For this review, take the finished solid that the model builds, in its own axes (mm). A direction names the side the tool comes from. Coordinates: 2 decimals unless noted, no trailing zeros. Loops run counter-clockwise (first coordinate to the right, second up) from the corner with the lowest first, then second, coordinate; pieces in that order, holes last. Notation, with made-up numbers: (-14, -35.75) -> (37, -35.75) arc R30 ccw to (37, -8.75) -> close; hole circle Ø4 at (16.25, 22.5). An arc over 180 degrees is marked (long way). One line per item, written item: value.
from build123d import *

# Parameters (mm, degrees)
SKETCH2_R                     = 4.7625
LOCATION_START                = -5.08
SKETCH4_R                     = 1.524
LOCATION_HOLE_OTHER_WAY_DEPTH = 81.074387678


with BuildPart() as part:
    # Handle: sweep along a path in Sketch3
    with BuildLine(Plane(origin=(0, 0, 0), x_dir=(1, 0, 0), z_dir=(0, 1, 0))) as handle_path:
        Line((62.70625, 19.05), (62.70625, -2.3495))
        ThreePointArc((62.70625, -2.3495), (57.814786799, -14.158536799), (46.00575, -19.05))
        Line((46.00575, -19.05), (-46.00575, -19.05))
        ThreePointArc((-46.00575, -19.05), (-57.814786799, -14.158536799), (-62.70625, -2.3495))
        Line((-62.70625, -2.3495), (-62.70625, 19.05))
    # Sketch2 → Handle (sweep)
    with BuildSketch(Plane.XY.offset(-19.05)):
        with Locations((-62.70625, 0)):
            Circle(SKETCH2_R)
    sweep(path=handle_path.line)

    # Location Hole cone 1 section (through the dimple's axis) → Location Hole (revolve, cut)
    with BuildSketch(Plane(origin=(-62.70625, 0, -13.97), x_dir=(0, 1, 0), z_dir=(1, 0, 0))):
        Polygon((0, 0), (1.524, 0), (0, 0.87988181), align=None)
    revolve(axis=Axis((-62.70625, 0, -13.97), (0, 0, 1)), mode=Mode.SUBTRACT)

    # Location Hole cone 2 section (through the dimple's axis) → Location Hole cone 2 (revolve, cut)
    with BuildSketch(Plane(origin=(62.70625, 0, -13.97), x_dir=(0, 1, 0), z_dir=(1, 0, 0))):
        Polygon((0, 0), (1.524, 0), (0, 0.87988181), align=None)
    revolve(axis=Axis((62.70625, 0, -13.97), (0, 0, 1)), mode=Mode.SUBTRACT)

    # Sketch4 → Location Hole other way (cut)
    with BuildSketch(Plane(origin=(0, 0, -19.05), x_dir=(-1, 0, 0), z_dir=(0, 0, -1)).offset(LOCATION_START)):
        with Locations((62.70625, 0)):
            Circle(SKETCH4_R)
        with Locations((-62.70625, 0)):
            Circle(SKETCH4_R)
    extrude(amount=LOCATION_HOLE_OTHER_WAY_DEPTH, mode=Mode.SUBTRACT)


solid = part.part
1. Insertion check: pin 1 Ø12 at (x, z) = (-21, 17.5) entering from -Y; pin 2 Ø4 at (x, y) = (62.71, 0) entering from +Z; pin 3 Ø3 at (y, z) = (-1, 18) entering from -X; pin 4 Ø4 at (y, z) = (-3, 15.5) entering from -X. Each pin has a flat end and moves straight along its axis. Give the tip position at first contact, or say it passes through.
Return value:
pin 1: stops at y = -4.76
pin 2: stops at z = 17.98
pin 3: stops at x = -62.05
pin 4: stops at x = -63.68
2. The part is to be moulded in two halves that separate along X. For faces 4 (the cylindrical face through (58.164, -1.431, -8.2)), 5 (the flat face through (-63, -2, -19.05)), say which applies: pulls with the +X half, pulls with the -X half, needs draft (parallel to the pull), parting line crosses it, or undercut.
Return value:
face 4: undercut
face 5: needs draft
3. To check wall thickness, follow probe 1 along X at (y, z) = (0, -17.25); probe 2 along X at (y, z) = (-0.5, -14); probe 3 along X at (y, z) = (3.5, -8). State the ranges of each line that lie inside material, in increasing order. Write a range as from..to.
Return value:
probe 1: x = -67.47..-64.23, -61.18..-57.94, 57.94..61.18, 64.23..67.47
probe 2: x = -67.44..-64.15, -61.27..-57.97, 57.97..61.27, 64.15..67.44
probe 3: x = -65.94..-59.48, 59.48..65.94
4. For faces 1 (the flat face through (63, -2, -19.05)), 2 (the cylindrical face through (-0.6, -1.4, 14.5)), 3 (the cylindrical face through (-58.164, -1.431, -8.5)), list the 3-axis set-ups (+Z, -Z, +X, -X, +Y, -Y) from which the entire face can be reached by the end or side of a thin tool; tool diameter is ignored.
Return value:
face 1: -Z, +X, -X, +Y, -Y
face 2: none
face 3: -Z
5. Take a section at B-B, the plane y = -3.25. Give the boundary of the cut face in (x, z).
Return value:
outline: (-66.19, -19.05) -> (-59.23, -19.05) -> (-59.23, 2.35) arc R13.22 cw to (-46.01, 15.57) -> (46.01, 15.57) arc R13.22 cw to (59.23, 2.35) -> (59.23, -19.05) -> (66.19, -19.05) -> (66.19, 2.35) arc R20.18 ccw to (46.01, 22.53) -> (-46.01, 22.53) arc R20.18 ccw to (-66.19, 2.35) -> close
